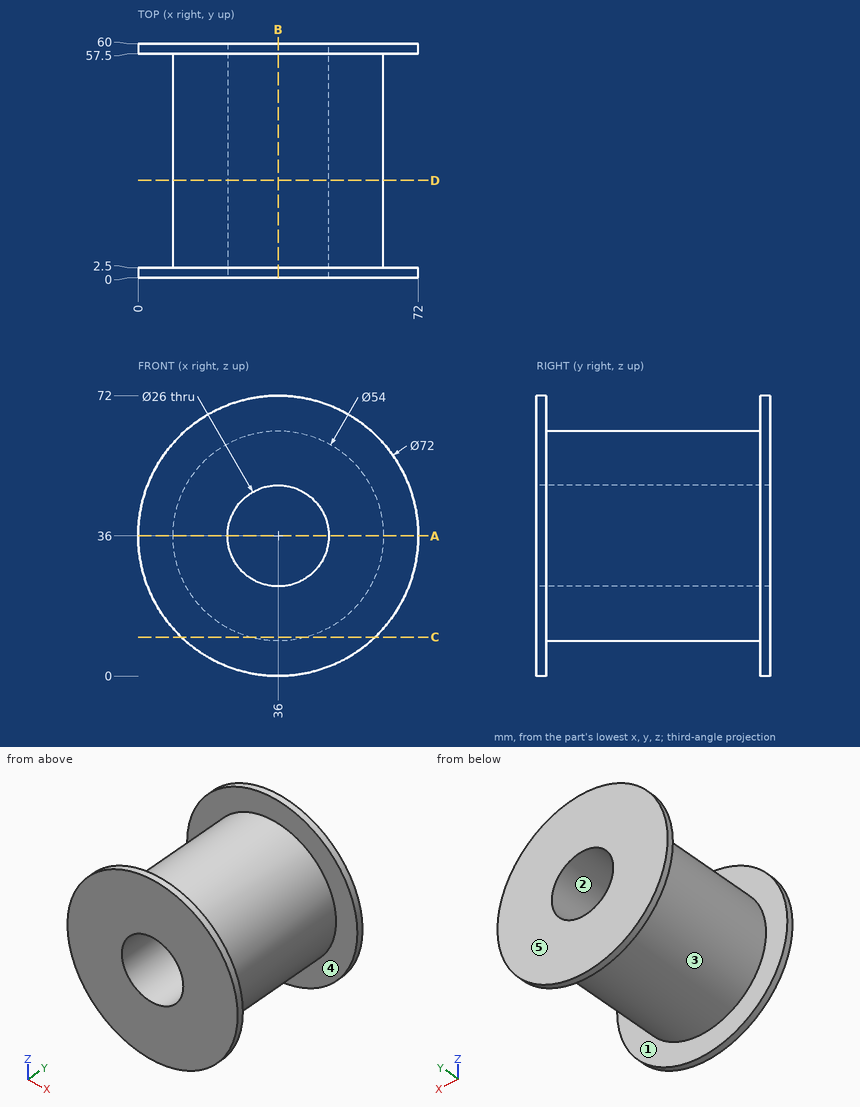
Answer from the drawing. Dimensions are ordinates in mm from the lowest x, y and z of the part. A direction names the side the tool comes from. Give positions to 0.01 mm unless a question says otherwise; leave off trailing zeros. Order: outer loops, then holes, each group sorted by start corner. A loop starts at its lowest first (then second) coordinate and runs counter-clockwise, first axis right, second up. Notation, with made-up numbers: (54.25, 23) -> (93.25, 23) arc R34 ccw to (93.25, 62) -> close; hole circle Ø11 at (7, 12.25). An arc over 180 degrees is marked (long way). Answer as a JSON object with one key per item and string values. Group by question number.
1. Section C-C on z = 10 is taken. Determine the outline of the cut face in (x, y).
2. Section A-A on z = 36 is taken. Determine the outline of the cut face in (x, y), plus the area to 3 significant figures.
3. Flat-ended cylindrical pins translate along their axes: pin 1 Ø1 at (y, z) = (48, 21.5) entering from -X; pin 2 Ø5 at (y, z) = (52, 51) entering from +X; pin 3 Ø5 at (x, y) = (43, 14.5) entering from +Z. Find the tip coordinate at first contact, or state that the pin passes through.
4. A tool of negligible diameter and unlimited length cuts with its end or side. For the marked faces 4 and 5, from which of +Z, -Z, +X, -X, +Y, -Y can it reach the whole face along a straight path? Write none if from no direction.
5. Consider line 1 along Y through (x, z) = (66, 28); line 2 along X through (y, z) = (4, 36.5); line 3 along Z through (x, y) = (36, 40). Determine where each line is inside the solid, lowest interval first. Write a range as [from, to].
6. The mould has two halves that part along X. Classify the marked faces 1, 2 and 3: released by +X, released by -X, zero draft, split by the parting line, or undercut.
7. Section D-D on y = 25 is taken. Determine the outline of the cut face in (x, z).
8. Section B-B on x = 36 is taken. Determine the outline of the cut face in (y, z), plus the area to 3 significant figures.
Result sheet:
{
 "1": {"outline": "(11.1, 0) -> (60.9, 0) -> (60.9, 2.5) -> (43.28, 2.5) -> (43.28, 57.5) -> (60.9, 57.5) -> (60.9, 60) -> (11.1, 60) -> (11.1, 57.5) -> (28.72, 57.5) -> (28.72, 2.5) -> (11.1, 2.5) -> close"},
 "2": {"outline": "(0, 0) -> (23, 0) -> (23, 60) -> (0, 60) -> (0, 57.5) -> (9, 57.5) -> (9, 2.5) -> (0, 2.5) -> close; (49, 0) -> (72, 0) -> (72, 2.5) -> (63, 2.5) -> (63, 57.5) -> (72, 57.5) -> (72, 60) -> (49, 60) -> close", "area": "1,770 mm^2"},
 "3": {"pin 1": "stops at x = 12.91", "pin 2": "stops at x = 59.93", "pin 3": "stops at z = 62.62"},
 "4": {"face 4": "none", "face 5": "+Z, -Z, +X, -X, +Y"},
 "5": {"line 1": "y = [0, 2.5], [57.5, 60]", "line 2": "x = [9, 23.01], [48.99, 63]", "line 3": "z = [9, 23], [49, 63]"},
 "6": {"face 1": "zero draft", "face 2": "undercut", "face 3": "split by the parting line"},
 "7": {"outline": "circle Ø54 at (36, 36); hole circle Ø26 at (36, 36)"},
 "8": {"outline": "(0, 0) -> (2.5, 0) -> (2.5, 9) -> (57.5, 9) -> (57.5, 0) -> (60, 0) -> (60, 23) -> (0, 23) -> close; (0, 49) -> (60, 49) -> (60, 72) -> (57.5, 72) -> (57.5, 63) -> (2.5, 63) -> (2.5, 72) -> (0, 72) -> close", "area": "1,770 mm^2"}
}
